Check sheet for the modelled part. Datum: model origin and axes. Units: mm. A direction names the side the tool comes from. Give positions to 0.01 mm unless a question says otherwise; leave off trailing zeros. Write each loop counter-clockwise with the first axis right and the second up, starting at its lowest first coordinate (ties: lowest second). Pieces come first, ordered by that corner, then holes. Notation, with made-up numbers: (22.5, -15) -> (54.5, -15) arc R18 cw to (54.5, 13) -> close; hole circle Ø7 at (66, 50). An arc over 180 degrees is marked (long way). Use a Markdown table: item, result. Add a question column.
1. Cross-section at B-B (z = 1.05). Enter the section's corners in (x, y), then the cut area to 3 significant figures.
2. Cross-section at A-A (x = 40). Enter the section's corners in (y, z), then the cut area to 3 significant figures.
3. Cross-section at C-C (y = 9.25). Enter the section's corners in (x, z), then the cut area to 3 significant figures.
4. Set-up check for faces 1 (the cylindrical face through (51.94, 14.41, 1.48)), 2 (the flat face through (33.805, 17.075, 1.521)): record each of +Z, -Z, +X, -X, +Y, -Y from which the full face is reachable in a straight line by a thin tool's end or side.
5. Scan lines: probe 1 along Y at (x, z) = (26, 2.05); probe 2 along Y at (x, z) = (35.5, 1.5); probe 3 along X at (y, z) = (12.5, 2.55). Record each from-to range of solid material in increasing order. Write a range as [from, to].
6. Gauge pin test, flat end, axial feed: P1, Ø1, axis at y = 10.5, z = 1.5, coming from the +X side. Record the tip position at first contact, or that the pin passes through.
from build123d import *

# Parameters (mm, degrees)
BOSS_EXTRUDE1_DEPTH = 3
CUT_EXTRUDE1_DEPTH  = 3
SKETCH3_R           = 1.55
CUT_EXTRUDE2_DEPTH  = 3
SKETCH4_R           = 1.55
CUT_EXTRUDE4_DEPTH  = 3
SKETCH5_R           = 1.55
CUT_EXTRUDE6_DEPTH  = 3


with BuildPart() as part:
    # Sketch1 → Boss-Extrude1 (new body)
    with BuildSketch(Plane.XY):
        with BuildLine():
            Line((-58.058617241, 24.191090517), (41.941382759, 24.191090517))
            ThreePointArc((41.941382759, 24.191090517), (51.941382759, 14.191090517), (41.941382759, 4.191090517))
            Line((41.941382759, 4.191090517), (-58.058617241, 4.191090517))
            ThreePointArc((-58.058617241, 4.191090517), (-68.058617241, 14.191090517), (-58.058617241, 24.191090517))
        make_face()
    extrude(amount=BOSS_EXTRUDE1_DEPTH)

    # Sketch2 → Cut-Extrude1 (cut)
    with BuildSketch(Plane.XY.offset(3)):
        with BuildLine():
            Line((41.520256561, 17.941090517), (25.870256561, 16.183590517))
            ThreePointArc((25.870256561, 16.183590517), (24.088990243, 14.191090517), (25.870256561, 12.198590517))
            Line((25.870256561, 12.198590517), (41.520256561, 10.441090517))
            ThreePointArc((41.520256561, 10.441090517), (45.714954976, 14.191090517), (41.520256561, 17.941090517))
        make_face()
    extrude(amount=-CUT_EXTRUDE1_DEPTH, mode=Mode.SUBTRACT)

    # Sketch3 → Cut-Extrude2 (cut)
    with BuildSketch(Plane.XY.offset(3)):
        with Locations((-58.058617241, 14.191090517)):
            Circle(SKETCH3_R)
    extrude(amount=-CUT_EXTRUDE2_DEPTH, mode=Mode.SUBTRACT)

    # Sketch4 → Cut-Extrude4 (cut)
    with BuildSketch(Plane(origin=(9.979459273, 1.433252018, 3), x_dir=(1, 0, 0), z_dir=(0, 0, 1))):
        with Locations((-4.038076514, 12.757838499)):
            Circle(SKETCH4_R)
    extrude(amount=-CUT_EXTRUDE4_DEPTH, mode=Mode.SUBTRACT)

    # Sketch5 → Cut-Extrude6 (cut)
    with BuildSketch(Plane(origin=(-9.979459273, 1.433252018, 0), x_dir=(-1, 0, 0), z_dir=(0, 0, -1))):
        with Locations((12.079157968, 12.757838499)):
            Circle(SKETCH5_R)
    extrude(amount=-CUT_EXTRUDE6_DEPTH, mode=Mode.SUBTRACT)


solid = part.part
Worked answers:
| question | item | result |
|---|---|---|
| 1 | outline | (-58.06, 4.19) -> (41.94, 4.19) arc R10 ccw to (41.94, 24.19) -> (-58.06, 24.19) arc R10 ccw to start; hole circle Ø3.1 at (-58.06, 14.19); hole circle Ø3.1 at (-22.06, 14.19); hole circle Ø3.1 at (5.94, 14.19); hole (25.87, 12.2) -> (41.52, 10.44) arc R3.77 ccw (long way) to (41.52, 17.94) -> (25.87, 16.18) arc R2.01 ccw to start |
| 1 | area | 2,170 mm² |
| 2 | outline | (4.19, 0) -> (10.61, 0) -> (10.61, 3) -> (4.19, 3) -> close; (17.77, 0) -> (24.19, 0) -> (24.19, 3) -> (17.77, 3) -> close |
| 2 | area | 38.5 mm² |
| 3 | outline | (-66.75, 0) -> (50.64, 0) -> (50.64, 3) -> (-66.75, 3) -> close |
| 3 | area | 352 mm² |
| 4 | face 1 | +Z, -Z, +X |
| 4 | face 2 | +Z, -Z |
| 5 | probe 1 | y = [4.19, 12.18], [16.2, 24.19] |
| 5 | probe 2 | y = [4.19, 11.12], [17.27, 24.19] |
| 5 | probe 3 | x = [-67.91, 25.02], [45.31, 51.8] |
| 6 | P1 | stops at x = 51.42 |
